```python
from build123d import *

# Parameters (mm, degrees)
SKETCH1_R                           = 28
BOSS_EXTRUDE1_DEPTH                 = 20.56
SKETCH2_R                           = 30.7
BOSS_EXTRUDE2_DEPTH                 = 70.12
SKETCH3_R                           = 28
BOSS_EXTRUDE3_DEPTH                 = 4.6
F_5_40_TAPPED_HOLE1_D               = 2.5781
F_5_40_TAPPED_HOLE1_ON_FACE_2_D     = 2.5781
F_5_40_TAPPED_HOLE1_ON_FACE_3_D     = 2.5781
M3X0_5_TAPPED_HOLE1_D               = 2.5
M3X0_5_TAPPED_HOLE1_DEPTH           = 7.5
M3X0_5_TAPPED_HOLE1_TIP             = 0.751075774
M3X0_5_TAPPED_HOLE1_ON_FACE_2_D     = 2.5
M3X0_5_TAPPED_HOLE1_ON_FACE_2_DEPTH = 7.5
M3X0_5_TAPPED_HOLE1_ON_FACE_2_TIP   = 0.751075774
FILLET1_R                           = 1


with BuildPart() as part:
    # Sketch1 → Boss-Extrude1 (new body)
    with BuildSketch(Plane.XY):
        Circle(SKETCH1_R)
    extrude(amount=BOSS_EXTRUDE1_DEPTH)

    # Sketch2 → Boss-Extrude2 (add)
    with BuildSketch(Plane.XY.offset(20.56)):
        Circle(SKETCH2_R)
    extrude(amount=BOSS_EXTRUDE2_DEPTH)

    # Sketch3 → Boss-Extrude3 (add)
    with BuildSketch(Plane.XY.offset(90.68)):
        Circle(SKETCH3_R)
    extrude(amount=BOSS_EXTRUDE3_DEPTH)

    # Sketch4 → Revolve1 (revolve)
    with BuildSketch(Plane(origin=(0, 0, 0), x_dir=(0, 0, -1), z_dir=(1, 0, 0)), mode=Mode.PRIVATE) as revolve1_sk:
        Polygon((-20.56, 30.7), (-20.56, 32), (-32.56, 32), (-35.56, 30.7), align=None)
        Polygon((-75.68, 30.7), (-90.68, 30.7), (-90.68, 32), (-78.68, 32), align=None)
    revolve(revolve1_sk.sketch.rotate(Axis((0, 0, 0), (0, 0, 1)), 90), axis=Axis((0, 0, 0), (0, 0, 1)))

    # #5-40 Tapped Hole1 (through all)
    with Locations(Plane(origin=(24.248711306, 14, 4.56), x_dir=(-0.5, 0.866025403784, 0), z_dir=(0.866025403784, 0.5, 0))):
        with Locations((0, 0)):
            Hole(F_5_40_TAPPED_HOLE1_D / 2)

    # #5-40 Tapped Hole1 on face 2 (through all)
    with Locations(Plane(origin=(-0.009573975, 27.999998363, 4.56), x_dir=(0.999999941518, 0.00034199998, 0), z_dir=(-0.00034199998, 0.999999941518, 0))):
        with Locations((0, 0)):
            Hole(F_5_40_TAPPED_HOLE1_ON_FACE_2_D / 2)

    # #5-40 Tapped Hole1 on face 3 (through all)
    with Locations(Plane(origin=(-24.248711306, 14, 4.56), x_dir=(-0.500000174844, -0.866025302838, 0), z_dir=(-0.866025302838, 0.500000174844, 0))):
        with Locations((0, 0)):
            Hole(F_5_40_TAPPED_HOLE1_ON_FACE_3_D / 2)

    # M3x0.5 Tapped Hole1
    with Locations(Plane(origin=(26.212865417, 18.354445963, 27.696295827), x_dir=(-0.573576436351, 0.819152044289, 0), z_dir=(0.819152044289, 0.573576436351, 0))):
        with Locations((0, 0)):
            Hole(M3X0_5_TAPPED_HOLE1_D / 2, depth=M3X0_5_TAPPED_HOLE1_DEPTH)
            with Locations((0, 0, -(M3X0_5_TAPPED_HOLE1_DEPTH + M3X0_5_TAPPED_HOLE1_TIP / 2))):  # 118° drill point
                Cone(0, M3X0_5_TAPPED_HOLE1_D / 2, M3X0_5_TAPPED_HOLE1_TIP, mode=Mode.SUBTRACT)

    # M3x0.5 Tapped Hole1 on face 2
    with Locations(Plane(origin=(-26.212865417, 18.354445963, 82), x_dir=(-0.573576164364, -0.819152234736, 0), z_dir=(-0.819152234736, 0.573576164364, 0))):
        with Locations((0, 0)):
            Hole(M3X0_5_TAPPED_HOLE1_ON_FACE_2_D / 2, depth=M3X0_5_TAPPED_HOLE1_ON_FACE_2_DEPTH)
            with Locations((0, 0, -(M3X0_5_TAPPED_HOLE1_ON_FACE_2_DEPTH + M3X0_5_TAPPED_HOLE1_ON_FACE_2_TIP / 2))):  # 118° drill point
                Cone(0, M3X0_5_TAPPED_HOLE1_ON_FACE_2_D / 2, M3X0_5_TAPPED_HOLE1_ON_FACE_2_TIP, mode=Mode.SUBTRACT)

    # Fillet1
    fillet1_edges = [part.edges().sort_by_distance(p)[0] for p in [
        (32, 0, 20.56),
        (32, 0, 90.68),
    ]]
    fillet(fillet1_edges, radius=FILLET1_R)


solid = part.part
```
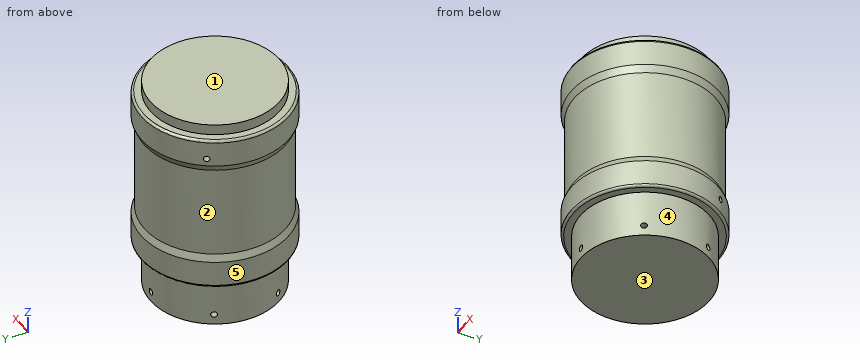
Design review of the part built by this model. Coordinates are the model's own, in mm. Face numbers are marked on the shaded views. A direction names the side the tool comes from. Give positions to 0.01 mm unless a question says otherwise; leave off trailing zeros. Write each loop counter-clockwise with the first axis right and the second up, starting at its lowest first coordinate (ties: lowest second). Pieces come first, ordered by that corner, then holes.
(1) Add section B-B (z = 87). Give the boundary of the cut face in (x, y), and give its area (3 significant figures).
Checked values:
outline: circle Ø64 at (0, 0)
area: 3,220 mm2
(2) Add section A-A (z = 4.56). Give the boundary of the cut face in (x, y), and give its area (3 significant figures).
Checked values:
outline: (-24.87, -12.87) - (-2.58, 0) - (-24.87, 12.87) arc R28 ccw to start; (-23.58, -15.1) arc R28 ccw to (-1.28, -27.97) - (-1.29, -2.23) - close; (-23.58, 15.1) - (-1.29, 2.23) - (-1.3, 27.97) arc R28 ccw to start; (1.28, 27.97) - (1.29, 2.23) - (23.58, 15.1) arc R28 ccw to start; (1.29, -2.23) - (1.3, -27.97) arc R28 ccw to (23.58, -15.1) - close; (2.58, 0) - (24.87, -12.87) arc R28 ccw to (24.87, 12.87) - close
area: 2,050 mm2
(3) Tool access review of the marked faces 4 and 5: name each direction out of +Z, -Z, +X, -X, +Y, -Y from which nothing blocks a thin tool from reaching the whole face with its end or side.
Checked values:
face 4: -Z
face 5: +Z, -Z
(4) Add section C-C (y = 4.5). Give the number of separate pieces and of enclosed holes in the cut face, and give its area (3 significant figures).
Checked values:
separate pieces: 1
enclosed holes: 3
area: 5,690 mm2
(5) Wall thickness on line 1 along X through (y, z) = (12, 4.56); line 2 along X through (y, z) = (8, 4); line 3 along Y through (x, z) = (-0.5, 22): over which ranges is each line inside the solid? List them lowest first.
Checked values:
line 1: x = -25.3 to -23.36, -18.21 to -1.29, 1.28 to 18.21, 23.36 to 25.3
line 2: x = -26.83 to -16.18, -11.53 to -1.16, 1.16 to 11.53, 16.18 to 26.83
line 3: y = -32 to 32
(6) Mouldability with a two-part tool opening along Z and no side actions: class the marked faces 1, 2 and 3 as +Z half, -Z half, draft (parallel to the pull), parting line (faces both ways), or undercut.
Checked values:
face 1: +Z half
face 2: undercut
face 3: -Z half
(7) Clearance check with flat-ended pins moving along their axes: pin 1 Ø10 at (x, z) = (13.5, 60.5) entering from -Y; pin 2 Ø6 at (y, z) = (6.5, 72.5) entering from +X; pin 3 Ø3.5 at (x, z) = (-0.05, 4.56) entering from +Y; pin 4 Ø8 at (x, y) = (-16, 24.5) entering from -Z. State where each tip first meets the part, or that it passes through.
Checked values:
pin 1: stops at y = -29.5
pin 2: stops at x = 30.5
pin 3: stops at y = 28
pin 4: stops at z = 0
